from build123d import *

# Parameters (mm, degrees)
BOSS_EXTRUDE1_DEPTH = 25.4
SKETCH3_R           = 6.35
CUT_EXTRUDE1_DEPTH  = 12.7
SKETCH4_R           = 3.556
CUT_EXTRUDE2_DEPTH  = 12.7
SKETCH11_R          = 4.6355
BOSS_EXTRUDE3_DEPTH = 2.032
CIRPATTERN1_COUNT   = 3
SKETCH12_R          = 2.0828
CUT_EXTRUDE4_DEPTH  = 2.9718
FILLET3_R           = 2.54


with BuildPart() as part:
    # Sketch1 → Boss-Extrude1 (new body)
    with BuildSketch(Plane(origin=(0, 0, 0), x_dir=(1, 0, 0), z_dir=(0, 1, 0))):
        Polygon((7.906621038, 9.792659833), (7.917579369, -9.673383406), (4.508232527, -11.732623201), (-12.391554014, -1.98820766), (-12.35878698, 1.994487054), (4.399412926, 11.682420986), align=None)
    extrude(amount=BOSS_EXTRUDE1_DEPTH)

    # Sketch3 → Cut-Extrude1 (cut)
    with BuildSketch(Plane(origin=(0, 25.4, 0), x_dir=(1, 0, 0), z_dir=(0, 1, 0))):
        Circle(SKETCH3_R)
    extrude(amount=-CUT_EXTRUDE1_DEPTH, mode=Mode.SUBTRACT)

    # Sketch4 → Cut-Extrude2 (cut)
    with BuildSketch(Plane.XZ):
        Circle(SKETCH4_R)
    extrude(amount=-CUT_EXTRUDE2_DEPTH, mode=Mode.SUBTRACT)

    # Sketch11 → Boss-Extrude3 (add, symmetric)
    with BuildSketch(Plane(origin=(-0.000811781, 0, 0.098668517), x_dir=(0.999966157, 0, 0.008227074), z_dir=(-0.008227074, 0, 0.999966157))):
        with BuildLine():
            Line((-12.151651157, 25.4), (-12.151651157, 0))
            Line((-12.151651157, 0), (-12.374777516, 0))
            ThreePointArc((-12.374777516, 0), (-14.579369049, 3.004291223), (-18.089777516, 4.2545))
            ThreePointArc((-18.089777516, 4.2545), (-26.535277516, 12.7), (-18.089777516, 21.1455))
            ThreePointArc((-18.089777516, 21.1455), (-14.579369049, 22.395708777), (-12.374777516, 25.4))
            Line((-12.374777516, 25.4), (-12.151651157, 25.4))
        make_face()
        with Locations((-18.089777516, 12.7)):
            Circle(SKETCH11_R, mode=Mode.SUBTRACT)
    boss_extrude3 = extrude(amount=BOSS_EXTRUDE3_DEPTH, both=True)

    # CirPattern1: Boss-Extrude3 ×3 about axis
    cirpattern1_axis = Axis((0, 0, 0), (0, 1, 0))
    for i in range(1, CIRPATTERN1_COUNT):
        add(boss_extrude3.rotate(cirpattern1_axis, i * 360 / CIRPATTERN1_COUNT))

    # Sketch12 → Cut-Extrude4 (cut)
    with BuildSketch(Plane(origin=(7.912131269, 0, -0.004454103), x_dir=(-0.000562946, 0, -0.999999842), z_dir=(0.999999842, 0, -0.000562946))):
        with Locations((0.010106248, 22.86)):
            Circle(SKETCH12_R)
    extrude(amount=-CUT_EXTRUDE4_DEPTH, mode=Mode.SUBTRACT)

    # Fillet3
    fillet3_edges = [part.edges().sort_by_distance(p)[0] for p in [
        (-12.320145535, 12.7, 2.029381784),
    ]]
    fillet(fillet3_edges, radius=FILLET3_R)


solid = part.part
Could you check a few things on this model? Use its own coordinates, in mm. A direction names the side the tool comes from. Coordinates: 2 decimals unless noted, no trailing zeros. Write each loop counter-clockwise with the first axis right and the second up, starting at its lowest first coordinate (ties: lowest second). Pieces come first, ordered by that corner, then holes. Notation, with made-up numbers: (44, 52) - (69, 52) arc R16 ccw to (69, 71) - close; hole circle Ø2 at (-31.75, 78). An arc over 180 degrees is marked (long way). Put each result on its own line as item: value. Start each with the question number.
Q1. I want a section at A-A on y = 14.5. Count the separate pieces of the cut face and the enclosed holes in it, plus the area to 3 significant figures.
Q2. I'm going to push flat-ended pins straight in: P1, Ø4, axis at y = 4.5, z = -14, coming from the +X side; P2, Ø3, axis at y = 19.5, z = -14, coming from the +X side; P3, Ø8, axis at y = 8.5, z = 18, coming from the +X side. Where does each tip first touch, or does it pass through?
Q3. Which directions (+Z, -Z, +X, -X, +Y, -Y) give clear straight access to the entire face, cutting with the end or side of a thin tool? Please do faces 1 (the cylindrical face through (-5.04, 19.14, 3.86)), 2 (the cylindrical face through (-12.334, 12.522, 2.115)), 3 (the flat face through (12.934, 10.056, 18.512)).
Q4. Thinking about a two-plate mould opening in Z: for faces 4 (the flat face through (3, 12.7, 3)), 5 (the cylindrical face through (7.31, 22.36, -12.67)), 6 (the flat face through (2.1, 25.4, 6.5)), which applies, pulls with the +Z half, pulls with the -Z half, needs draft (parallel to the pull), parting line crosses it, or undercut?
Q5. Please list where these lines run through material, in increasing order: L1, parallel to Z at x = 3.5, y = 18; L2, parallel to Z at x = 2, y = 6.5; L3, parallel to X at y = 17.5, z = 0.
Q6. I want a section at B-B on x = 0. Write out the boundary of the cut face in (y, z), plus the area to 3 significant figures.
Checks:
1. separate pieces: 4
1. enclosed holes: 1
1. area: 244 mm²
2. P1: x = 11.66
2. P2: x = 11.36
2. P3: x = 14.73
3. face 1: +Y
3. face 2: +Z, -X, +Y, -Y
3. face 3: +X, +Y, -Y
4. face 4: undercut
4. face 5: pulls with the -Z half
4. face 6: needs draft
5. L1: -11.16 to -5.3, 5.3 to 11.15
5. L2: -10.3 to -2.94, 2.94 to 10.29
5. L3: -25.04 to -6.35, 6.35 to 7.91
6. outline: (0, -9.14) - (25.4, -9.14) - (25.4, -6.35) - (12.7, -6.35) - (12.7, -3.56) - (0, -3.56) - close; (0, 3.56) - (12.7, 3.56) - (12.7, 6.35) - (25.4, 6.35) - (25.4, 9.13) - (0, 9.13) - close
6. area: 213 mm²
